from build123d import *

# Parameters (mm, degrees)
SKETCH1_W           = 7.2
SKETCH1_H           = 39
SKETCH1_R           = 1.5
BOSS_EXTRUDE1_DEPTH = 1.2
SKETCH2_W           = 1.2
SKETCH2_H           = 39
BOSS_EXTRUDE2_DEPTH = 6
CUT_EXTRUDE1_REACH  = 3.2
SKETCH3_R           = 1.5


with BuildPart() as part:
    # Sketch1 → Boss-Extrude1 (new body)
    with BuildSketch(Plane.XY):
        Rectangle(SKETCH1_W, SKETCH1_H)
        with Locations((0, -5)):
            Circle(SKETCH1_R, mode=Mode.SUBTRACT)
        with Locations((0, -15)):
            Circle(SKETCH1_R, mode=Mode.SUBTRACT)
        with Locations((0, 15)):
            Circle(SKETCH1_R, mode=Mode.SUBTRACT)
        with Locations((0, 5)):
            Circle(SKETCH1_R, mode=Mode.SUBTRACT)
    extrude(amount=BOSS_EXTRUDE1_DEPTH)

    # Sketch2 → Boss-Extrude2 (add)
    with BuildSketch(Plane.XY.offset(1.2)):
        with Locations((3, 0)):
            Rectangle(SKETCH2_W, SKETCH2_H)
    extrude(amount=BOSS_EXTRUDE2_DEPTH)

    # Sketch3 → Cut-Extrude1 (cut, up to next)
    with BuildSketch(Plane.ZY.offset(-2.4), mode=Mode.PRIVATE) as cut_extrude1_sk1:
        with Locations((4.2, 15)):
            Circle(SKETCH3_R)
    cut_extrude1_tool1 = extrude(cut_extrude1_sk1.sketch, amount=-CUT_EXTRUDE1_REACH, mode=Mode.PRIVATE) & part.part
    add(cut_extrude1_tool1.solids().sort_by_distance((2.4, 15, 4.2))[0], mode=Mode.SUBTRACT)
    # Sketch3 → Cut-Extrude1 (cut, up to next)
    with BuildSketch(Plane.ZY.offset(-2.4), mode=Mode.PRIVATE) as cut_extrude1_sk2:
        with Locations((4.2, 5)):
            Circle(SKETCH3_R)
    cut_extrude1_tool2 = extrude(cut_extrude1_sk2.sketch, amount=-CUT_EXTRUDE1_REACH, mode=Mode.PRIVATE) & part.part
    add(cut_extrude1_tool2.solids().sort_by_distance((2.4, 5, 4.2))[0], mode=Mode.SUBTRACT)
    # Sketch3 → Cut-Extrude1 (cut, up to next)
    with BuildSketch(Plane.ZY.offset(-2.4), mode=Mode.PRIVATE) as cut_extrude1_sk3:
        with Locations((4.2, -5)):
            Circle(SKETCH3_R)
    cut_extrude1_tool3 = extrude(cut_extrude1_sk3.sketch, amount=-CUT_EXTRUDE1_REACH, mode=Mode.PRIVATE) & part.part
    add(cut_extrude1_tool3.solids().sort_by_distance((2.4, -5, 4.2))[0], mode=Mode.SUBTRACT)
    # Sketch3 → Cut-Extrude1 (cut, up to next)
    with BuildSketch(Plane.ZY.offset(-2.4), mode=Mode.PRIVATE) as cut_extrude1_sk4:
        with Locations((4.2, -15)):
            Circle(SKETCH3_R)
    cut_extrude1_tool4 = extrude(cut_extrude1_sk4.sketch, amount=-CUT_EXTRUDE1_REACH, mode=Mode.PRIVATE) & part.part
    add(cut_extrude1_tool4.solids().sort_by_distance((2.4, -15, 4.2))[0], mode=Mode.SUBTRACT)


solid = part.part
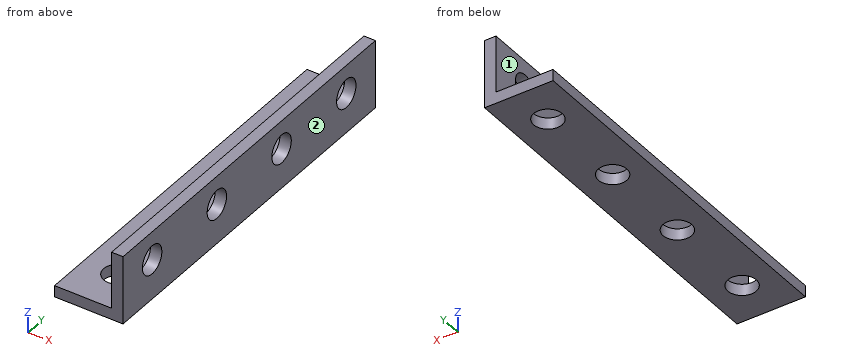
CAD build for the part. Positions are in the model's coordinates, mm. Face numbers are marked on the shaded views. A direction names the side the tool comes from. Give positions to 0.01 mm unless a question says otherwise; leave off trailing zeros. Write each loop counter-clockwise with the first axis right and the second up, starting at its lowest first coordinate (ties: lowest second). Pieces come first, ordered by that corner, then holes. Notation, with made-up numbers: M 68,69 L 121,69 A22 ccw 121,90 Z; hole C -32,41.5 d8. An arc over 180 degrees is marked long. Put each result on its own line as item: value. Start each with the question number.
(1) Probe L1, parallel to Y at x = 0, z = 0.95; L2, parallel to X at y = 6.5, z = 5; L3, parallel to Z at x = -1.5, y = -7.5. List the from-to ranges inside material, lowest first.
(2) Band-saw the part on A-A, the plane x = 0. Write the cut outline in (y, z), and give its area (3 significant figures).
(3) Band-saw the part on D-D, the plane x = -2.5. Write the cut outline in (y, z), and give its area (3 significant figures).
(4) Band-saw the part on B-B, the plane z = 4.2. Write the cut outline in (x, y), and give its area (3 significant figures).
(5) Which spindle directions (+Z, -Z, +X, -X, +Y, -Y) get a long thin tool onto all of the face, cutting with end or side? Do the marked faces 1 and 2. Say none if no direction does.
(6) Band-saw the part on C-C, the plane y = -15. Write the cut outline in (x, z), and give its area (3 significant figures).
(7) Flat gauge pins, fed straight in: pin 1 Ø2.5 at (x, y) = (0, 5) entering from -Z; pin 2 Ø1.5 at (y, z) = (-4.5, 5) entering from +X; pin 3 Ø4 at (y, z) = (-15, 4.2) entering from -X. Where does each tip first touch, or does it go through?
Response values:
1. L1: y = -19.5 to -16.5, -13.5 to -6.5, -3.5 to 3.5, 6.5 to 13.5, 16.5 to 19.5
1. L2: x = 2.4 to 3.6
1. L3: z = 0 to 1.2
2. outline: M -19.5,0 L -16.5,0 L -16.5,1.2 L -19.5,1.2 Z; M -13.5,0 L -6.5,0 L -6.5,1.2 L -13.5,1.2 Z; M -3.5,0 L 3.5,0 L 3.5,1.2 L -3.5,1.2 Z; M 6.5,0 L 13.5,0 L 13.5,1.2 L 6.5,1.2 Z; M 16.5,0 L 19.5,0 L 19.5,1.2 L 16.5,1.2 Z
2. area: 32.4 mm2
3. outline: M -19.5,0 L 19.5,0 L 19.5,1.2 L -19.5,1.2 Z
3. area: 46.8 mm2
4. outline: M 2.4,-19.5 L 3.6,-19.5 L 3.6,-16.5 L 2.4,-16.5 Z; M 2.4,-13.5 L 3.6,-13.5 L 3.6,-6.5 L 2.4,-6.5 Z; M 2.4,-3.5 L 3.6,-3.5 L 3.6,3.5 L 2.4,3.5 Z; M 2.4,6.5 L 3.6,6.5 L 3.6,13.5 L 2.4,13.5 Z; M 2.4,16.5 L 3.6,16.5 L 3.6,19.5 L 2.4,19.5 Z
4. area: 32.4 mm2
5. face 1: +Z, -X, +Y, -Y
5. face 2: +Z, -Z, +X, +Y, -Y
6. outline: M -3.6,0 L -1.5,0 L -1.5,1.2 L -3.6,1.2 Z; M 1.5,0 L 3.6,0 L 3.6,2.7 L 2.4,2.7 L 2.4,1.2 L 1.5,1.2 Z; M 2.4,5.7 L 3.6,5.7 L 3.6,7.2 L 2.4,7.2 Z
6. area: 8.64 mm2
7. pin 1: passes through
7. pin 2: stops at x = 3.6
7. pin 3: stops at x = 2.4
